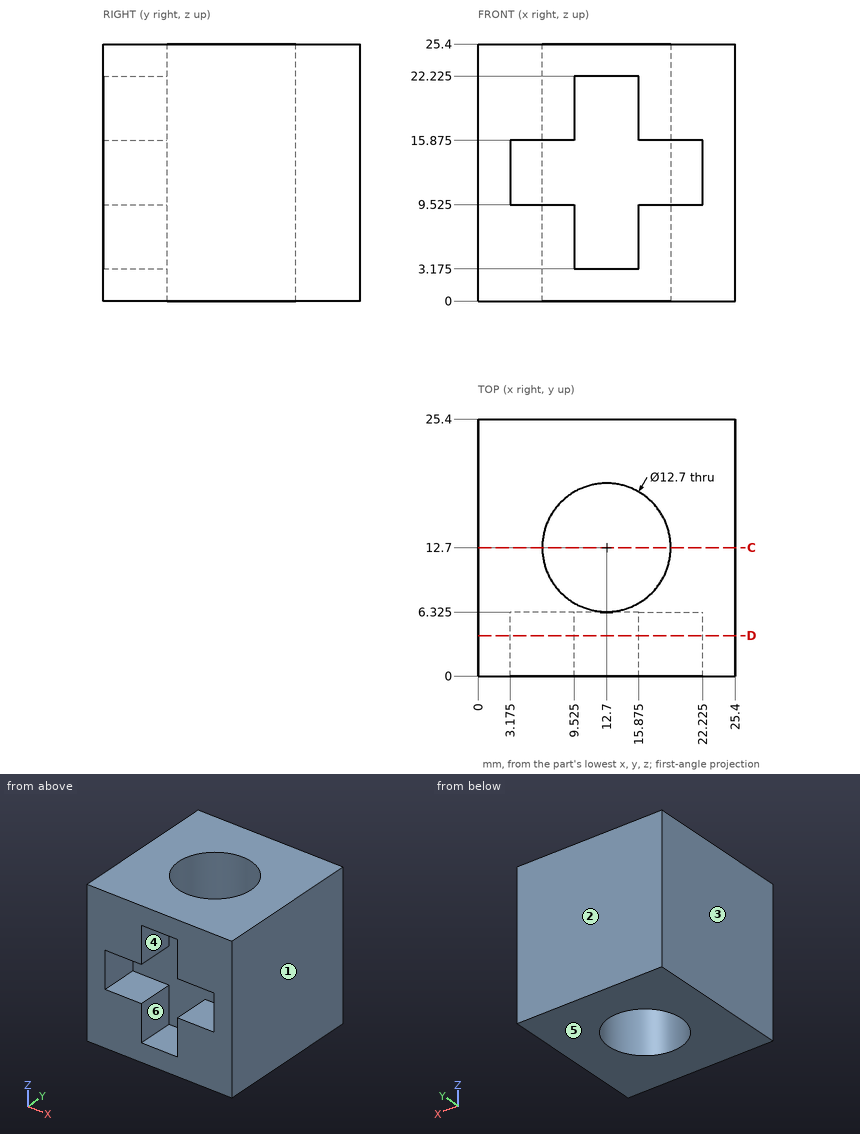
The drawing under review shows one solid part. Ordinate dimensions are in mm from its lowest x, y, z. A direction names the side the tool comes from. Round coordinates to 2 decimals unless told otherwise and drop trailing zeros. Loops run counter-clockwise (first coordinate to the right, second up) from the corner with the lowest first, then second, coordinate; pieces in that order, holes last. Notation, with made-up numbers: (-24, -8.75) -> (-15, -8.75) arc R12 cw to (-15, 12.25) -> close; hole circle Ø8 at (75.25, 19). An arc over 180 degrees is marked (long way). One line per question, with ' | ' between items. Start each with the question number.
Item 1: Machinability: for the marked faces 5 and 6, which of the approach directions +Z, -Z, +X, -X, +Y, -Y give a long, thin tool a straight path to every point of the face, cutting with its end or side? Answer none if there is none.
Item 2: Add section C-C, the plane y = 12.7. Write out the cut boundary in (x, z).
Item 3: Wall thickness on line 1 along X through (y, z) = (5, 3.5) (1 decimal); line 2 along X through (y, z) = (14.75, 19): over which ranges is each line inside the solid? List them lowest first. Write a range as [from, to].
Item 4: Draft analysis for pull direction X (two halves, no side actions). For the marked faces 1, 2, 3 and 4, state which applies: +X half, -X half, draft (parallel to the pull), parting line (faces both ways), or undercut.
Item 5: Add section D-D, the plane y = 4. Write out the cut boundary in (x, z) (1 decimal).
Return value:
1) face 5: -Z, +X, -X, +Y, -Y | face 6: -Y
2) outline: (0, 0) -> (6.35, 0) -> (6.35, 25.4) -> (0, 25.4) -> close; (19.05, 0) -> (25.4, 0) -> (25.4, 25.4) -> (19.05, 25.4) -> close
3) line 1: x = [0, 9.5], [15.9, 25.4] | line 2: x = [0, 6.69], [18.71, 25.4]
4) face 1: +X half | face 2: draft | face 3: -X half | face 4: undercut
5) outline: (0, 0) -> (25.4, 0) -> (25.4, 25.4) -> (0, 25.4) -> close; hole (3.2, 9.5) -> (9.5, 9.5) -> (9.5, 3.2) -> (15.9, 3.2) -> (15.9, 9.5) -> (22.2, 9.5) -> (22.2, 15.9) -> (15.9, 15.9) -> (15.9, 22.2) -> (9.5, 22.2) -> (9.5, 15.9) -> (3.2, 15.9) -> close
